The model under review builds one solid part; all positions refer to its coordinate system, in mm. A direction names the side the tool comes from. Round coordinates to 2 decimals unless told otherwise and drop trailing zeros. Write each loop counter-clockwise with the first axis right and the second up, starting at its lowest first coordinate (ties: lowest second). Pieces come first, ordered by that corner, then holes. Notation, with made-up numbers: M 66.25,28.5 L 110.25,28.5 A20 ccw 110.25,42.5 Z; hole C -22.5,24.25 d2. An arc over 180 degrees is marked long. One line per item, written item: value. Start each with the question number.
1) For P1, Ø1.5, axis at x = 22.5, y = -8.5, coming from the +Z side; P2, Ø11, axis at y = -29.5, z = 13.5, coming from the +X side; P3, Ø12, axis at x = 1.5, y = -32.5, coming from the +Z side, all flat-tipped, find the tip position at first contact; note any pin that passes through.
2) Take a section at B-B, the plane x = 29.5. Write out the cut boundary in (y, z).
3) Take a section at D-D, the plane y = 20.5. Write out the cut boundary in (x, z), and give its area (3 significant figures).
4) Tool access review of faces 5 (the face through (21, -22.327, 13)), 6 (the face through (28, 10.741, 104)), 7 (the face through (0.762, -34, 11)), 8 (the face through (29, -34, 25.604)), 9 (the face through (-35, -7, 22.352)): name each direction out of +Z, -Z, +X, -X, +Y, -Y from which nothing blocks a thin tool from reaching the whole face with its end or side.
5) Take a section at C-C, the plane y = -37.5. Write out the cut boundary in (x, z).
6) Mouldability with a two-part tool opening along Y and no side actions: class faces 1 (the face through (28, 20, 124.714)), 2 (the face through (-23, -45.374, 11)), 3 (the face through (17, 29.441, 48)), 4 (the face through (28, -26.673, 104)) as +Y half, -Y half, draft (parallel to the pull), parting line (faces both ways), or undercut.
7) Take a section at A-A, the plane z = 76.5. Write out the cut boundary in (x, y), and give its area (3 significant figures).
8) Wall thickness on probe 1 along X at (y, z) = (23, 103.5); probe 2 along Z at (x, y) = (-45.5, 12); probe 3 along Z at (x, y) = (22.5, -36): over which ranges is each line inside the solid? List them lowest first.
from build123d import *

# Parameters (mm, degrees)
F1_DEPTH = 124.714
F3_DEPTH = 102.362
F5_DEPTH = 25.4
F6_W     = 23.046266
F6_H     = 25.604162
F7_DEPTH = 39.878


with BuildPart() as f1:
    # F0 (on Top) → F1 (new body)
    with BuildSketch(Plane.XY):
        with BuildLine():
            Line((40.64, 29.44091), (-46.874546, 29.44091))
            ThreePointArc((-46.874546, 29.44091), (-84.281819, -7.966364), (-46.874546, -45.373637))
            Line((-46.874546, -45.373637), (40.64, -45.373637))
            Line((40.64, -45.373637), (40.64, 29.44091))
        make_face()
    extrude(amount=F1_DEPTH)

    # F2 (on face) → F3 (cut)
    with BuildSketch(Plane.XY.offset(124.714)):
        with BuildLine():
            Line((16.18675, -45.373637), (16.18675, 29.44091))
            Line((16.18675, 29.44091), (-46.874546, 29.44091))
            ThreePointArc((-46.874546, 29.44091), (-84.281819, -7.966364), (-46.874546, -45.373637))
            Line((-46.874546, -45.373637), (16.18675, -45.373637))
        make_face()
    extrude(amount=-F3_DEPTH, mode=Mode.SUBTRACT)

    # F4 (on face) → F5 (cut)
    with BuildSketch(Plane(origin=(16.18675, 0, 0), x_dir=(0, -1, 0), z_dir=(-1, 0, 0))):
        with BuildLine():
            Line((26.673464, 124.714), (-10.740736, 124.714))
            Line((-10.740736, 124.714), (-10.740736, 83.048187))
            ThreePointArc((-10.740736, 83.048187), (7.966364, 64.341087), (26.673464, 83.048187))
            Line((26.673464, 83.048187), (26.673464, 124.714))
        make_face()
    extrude(amount=-F5_DEPTH, mode=Mode.SUBTRACT)

    # F6 (on face) → F7 (cut)
    with BuildSketch(Plane.YZ.offset(40.64)):
        with Locations((-33.850504, 12.802081)):
            Rectangle(F6_W, F6_H)
    extrude(amount=-F7_DEPTH, mode=Mode.SUBTRACT)


solid = f1.part
Checked values:
1. P1: stops at z = 64.39
1. P2: stops at x = 0.76
1. P3: stops at z = 22.35
2. outline: M -45.37,25.6 L -22.33,25.6 L -22.33,0 L 29.44,0 L 29.44,124.71 L 10.74,124.71 L 10.74,83.05 A18.71 cw -26.67,83.05 L -26.67,124.71 L -45.37,124.71 Z
3. outline: M -71.14,0 L 40.64,0 L 40.64,124.71 L 16.19,124.71 L 16.19,22.35 L -71.14,22.35 Z
3. area: 5,000 mm2
4. face 5: -Z, +X, -Y
4. face 6: +Z, +X, -X
4. face 7: +Z, -Z, +X, -Y
4. face 8: -Z, +X, -X, -Y
4. face 9: +Z, -X, +Y, -Y
5. outline: M -69.83,0 L 0.76,0 L 0.76,22.35 L -69.83,22.35 Z; M 16.19,25.6 L 40.64,25.6 L 40.64,124.71 L 16.19,124.71 Z
6. face 1: draft
6. face 2: -Y half
6. face 3: +Y half
6. face 4: undercut
7. outline: M 16.19,-45.37 L 40.64,-45.37 L 40.64,-25.49 L 16.19,-25.49 Z; M 16.19,9.56 L 40.64,9.56 L 40.64,29.44 L 16.19,29.44 Z
7. area: 972 mm2
8. probe 1: x = 16.19 to 40.64
8. probe 2: z = 0 to 22.35
8. probe 3: z = 25.6 to 124.71
